from build123d import *
from OCP.BRepFilletAPI import BRepFilletAPI_MakeChamfer

# Parameters (mm, degrees)
BOSS_EXTRUDE1_DEPTH = 15
CHAMFER1_SIZE       = 10
CHAMFER1_SIZE2      = 10.462732323
CHAMFER1_SIZE2_2    = 9.593689253
CHAMFER2_SIZE       = 20
CHAMFER2_SIZE2      = 23.221000733
CHAMFER2_SIZE2_2    = 17.830293244


with BuildPart() as part:
    # Sketch2 → Boss-Extrude1 (new body)
    with BuildSketch(Plane(origin=(0, 0, 0), x_dir=(1, 0, 0), z_dir=(0, 1, 0))):
        Polygon((197.980321351, 0), (217.75302006, -150.572975632), (172.735338859, -150.572975632), (171.432941589, -135.629642818), (156.489589987, -136.932041726), (157.678475714, -150.572975632), (-157.678475714, -150.572975632), (-156.489589987, -136.932041726), (-171.432941589, -135.629642818), (-172.735338859, -150.572975632), (-217.75302006, -150.572975632), (-197.980321351, 0), align=None)
        Polygon((108.492166043, -45.171892689), (110.449460378, -90.343785379), (-110.449460378, -90.343785379), (-108.492166043, -45.171892689), align=None, mode=Mode.SUBTRACT)
        Polygon((-163.549029189, -45.171892689), (-167.372507504, -89.041386471), (-152.429155902, -90.343785379), (-148.605677588, -46.474291597), align=None, mode=Mode.SUBTRACT)
        Polygon((152.429155902, -90.343785379), (148.605677588, -46.474291597), (163.549029189, -45.171892689), (167.372507504, -89.041386471), align=None, mode=Mode.SUBTRACT)
    extrude(amount=-BOSS_EXTRUDE1_DEPTH)

    # Chamfer1: one chamfer whose edges measure the first distance from different faces: ONE call of the kernel's chamfer builder (chamfer() names one face for all edges)
    chamfer1_edges_1 = [part.edges().sort_by_distance(p)[0] for p in [
        (-108.492166043, -7.5, 45.171892689),
    ]]
    chamfer1_side_1 = [part.faces().sort_by_distance(p)[0] for p in [
        (0, -7.5, 45.171892689),
    ]]
    chamfer1_edges_2 = [part.edges().sort_by_distance(p)[0] for p in [
        (108.492166043, -7.5, 45.171892689),
    ]]
    chamfer1_side_2 = [part.faces().sort_by_distance(p)[0] for p in [
        (109.470813211, -7.5, 67.757839034),
    ]]
    chamfer1_edges_3 = [part.edges().sort_by_distance(p)[0] for p in [
        (110.449460378, -7.5, 90.343785379),
    ]]
    chamfer1_side_3 = [part.faces().sort_by_distance(p)[0] for p in [
        (0, -7.5, 90.343785379),
    ]]
    chamfer1_edges_4 = [part.edges().sort_by_distance(p)[0] for p in [
        (-110.449460378, -7.5, 90.343785379),
    ]]
    chamfer1_side_4 = [part.faces().sort_by_distance(p)[0] for p in [
        (-109.470813211, -7.5, 67.757839034),
    ]]
    chamfer1 = BRepFilletAPI_MakeChamfer(part.part.solid().wrapped)
    for e in chamfer1_edges_1:
        chamfer1.Add(CHAMFER1_SIZE, CHAMFER1_SIZE2, e.wrapped, chamfer1_side_1[0].wrapped)  # the first distance lies on this face
    for e in chamfer1_edges_2:
        chamfer1.Add(CHAMFER1_SIZE, CHAMFER1_SIZE2, e.wrapped, chamfer1_side_2[0].wrapped)  # the first distance lies on this face
    for e in chamfer1_edges_3:
        chamfer1.Add(CHAMFER1_SIZE, CHAMFER1_SIZE2_2, e.wrapped, chamfer1_side_3[0].wrapped)  # the first distance lies on this face
    for e in chamfer1_edges_4:
        chamfer1.Add(CHAMFER1_SIZE, CHAMFER1_SIZE2_2, e.wrapped, chamfer1_side_4[0].wrapped)  # the first distance lies on this face
    add(Compound.cast(chamfer1.Shape()), mode=Mode.REPLACE)

    # Chamfer2: one chamfer whose edges measure the first distance from different faces: ONE call of the kernel's chamfer builder (chamfer() names one face for all edges)
    chamfer2_edges_1 = [part.edges().sort_by_distance(p)[0] for p in [
        (197.980321351, -7.5, 0),
    ]]
    chamfer2_side_1 = [part.faces().sort_by_distance(p)[0] for p in [
        (0, -7.5, 0),
    ]]
    chamfer2_edges_2 = [part.edges().sort_by_distance(p)[0] for p in [
        (217.75302006, -7.5, 150.572975632),
    ]]
    chamfer2_side_2 = [part.faces().sort_by_distance(p)[0] for p in [
        (207.866670706, -7.5, 75.286487816),
    ]]
    chamfer2_edges_3 = [part.edges().sort_by_distance(p)[0] for p in [
        (-217.75302006, -7.5, 150.572975632),
    ]]
    chamfer2_side_3 = [part.faces().sort_by_distance(p)[0] for p in [
        (-195.24417946, -7.5, 150.572975632),
    ]]
    chamfer2_edges_4 = [part.edges().sort_by_distance(p)[0] for p in [
        (-197.980321351, -7.5, 0),
    ]]
    chamfer2_side_4 = [part.faces().sort_by_distance(p)[0] for p in [
        (-207.866670706, -7.5, 75.286487816),
    ]]
    chamfer2 = BRepFilletAPI_MakeChamfer(part.part.solid().wrapped)
    for e in chamfer2_edges_1:
        chamfer2.Add(CHAMFER2_SIZE, CHAMFER2_SIZE2, e.wrapped, chamfer2_side_1[0].wrapped)  # the first distance lies on this face
    for e in chamfer2_edges_2:
        chamfer2.Add(CHAMFER2_SIZE, CHAMFER2_SIZE2_2, e.wrapped, chamfer2_side_2[0].wrapped)  # the first distance lies on this face
    for e in chamfer2_edges_3:
        chamfer2.Add(CHAMFER2_SIZE, CHAMFER2_SIZE2_2, e.wrapped, chamfer2_side_3[0].wrapped)  # the first distance lies on this face
    for e in chamfer2_edges_4:
        chamfer2.Add(CHAMFER2_SIZE, CHAMFER2_SIZE2, e.wrapped, chamfer2_side_4[0].wrapped)  # the first distance lies on this face
    add(Compound.cast(chamfer2.Shape()), mode=Mode.REPLACE)


solid = part.part
Model file for the job. Use its own axes, mm. A direction names the side the tool comes from. Coordinates: 2 decimals unless noted, no trailing zeros. Write each loop counter-clockwise with the first axis right and the second up, starting at its lowest first coordinate (ties: lowest second). Pieces come first, ordered by that corner, then holes. Notation, with made-up numbers: (-17.75, 51.25) -> (-12.75, 51.25) arc R23 ccw to (-12.75, 78.25) -> close; hole circle Ø3 at (54.5, 6). An arc over 180 degrees is marked (long way). One line per item, written item: value. Start each with the question number.
1) Flat gauge pins, fed straight in: pin 1 Ø4 at (y, z) = (-3.5, 135) entering from -X; pin 2 Ø3 at (y, z) = (-10.5, 39.5) entering from -X. Where does each tip first touch, or does it go through?
2) Probe probe 1 along X at (y, z) = (-1, 82); probe 2 along X at (y, z) = (-4.25, 141); probe 3 along Z at (x, y) = (93, -6.5). List the from-to ranges inside material, lowest first.
3) Slice it at B-B on x = 59.5. Write the cut outline in (y, z).
4) Pull direction X, two halves, no side cores. Call faces 4 (the face through (-1, -7, 0)), 5 (the face through (189.65, -7.4, 11.67)), 6 (the face through (165.434, -7.395, 66.8)): +X half, -X half, draft (parallel to the pull), parting line (faces both ways), or undercut.
5) Slice it at A-A on y = -12.75. Count the separate pieces of the cut face and the enclosed holes in it, then the cut area to 3 significant figures.
6) Slice it at D-D on z = 94.5. Write the cut outline in (x, y).
7) Slice it at C-C on z = 38. Write the cut outline in (x, y).
8) Which spindle directions (+Z, -Z, +X, -X, +Y, -Y) get a long thin tool onto all of the face, cutting with end or side? Do faces 1 (the face through (-155.973, -7.395, 45.832)), 2 (the face through (172.093, -7.395, 143.206)), 3 (the face through (2, -7, 150.573)). Say none if no direction does.
Answers follow:
1. pin 1: x = -215.33
1. pin 2: x = -203.36
2. probe 1: -208.75 to -166.76, -151.7 to -108.51, 108.79 to 151.7, 166.76 to 208.75
2. probe 2: -207.33 to -171.9, -156.84 to 156.84, 171.9 to 207.27
2. probe 3: 0 to 45.17, 90.34 to 150.57
3. outline: (-15, 0) -> (0, 0) -> (0, 45.17) -> (-15, 45.17) -> close; (-15, 90.34) -> (0, 90.34) -> (0, 150.57) -> (-15, 150.57) -> close
4. face 4: draft
4. face 5: +X half
4. face 6: undercut
5. separate pieces: 1
5. enclosed holes: 3
5. area: 50,300 mm2
6. outline: (-210.39, -15) -> (210.39, -15) -> (210.39, 0) -> (-210.39, 0) -> close
7. outline: (-202.97, -15) -> (202.97, -15) -> (202.97, 0) -> (-202.97, 0) -> close
8. face 1: +Y, -Y
8. face 2: +Z, +Y, -Y
8. face 3: +Z, +X, -X, +Y, -Y
